Input: part model. Units: mm. Frame: model coordinates. Face numbers are marked on the shaded views. A direction names the side the tool comes from. Coordinates: 2 decimals unless noted, no trailing zeros.
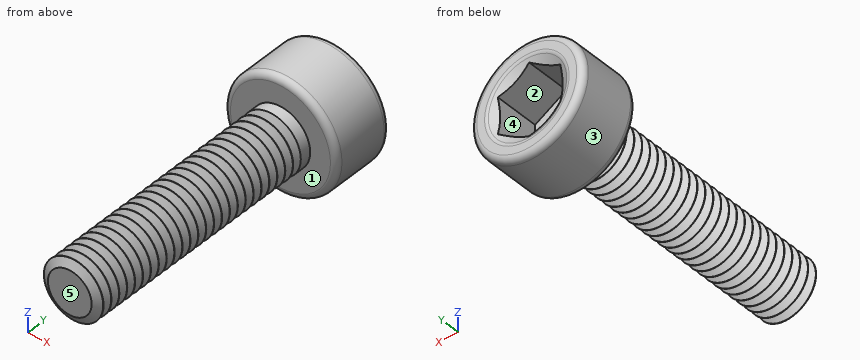
```python
from build123d import *

# Parameters (mm, degrees)
CUT_EXTRUDE1_DEPTH = 1.5
SKETCH3_R          = 1.3
CUT_EXTRUDE2_DEPTH = 1
CUT_EXTRUDE2_DRAFT = -60
FILLET1_R          = 0.2
LPATTERN1_COUNT    = 26
LPATTERN1_PITCH    = 0.3


with BuildPart() as part:
    # Sketch1 → Revolve1 (revolve)
    with BuildSketch(Plane.XY):
        with BuildLine():
            Line((0, 2), (0, -8))
            Line((0, -8), (0.95, -8))
            Line((0.95, -8), (0.95, 0))
            Line((0.95, 0), (1.6, 0))
            ThreePointArc((1.6, 0), (1.741421356, 0.058578644), (1.8, 0.2))
            Line((1.8, 0.2), (1.8, 1.8))
            ThreePointArc((1.8, 1.8), (1.741421356, 1.941421356), (1.6, 2))
            Line((1.6, 2), (0, 2))
        make_face()
    revolve(axis=Axis((0, 2, 0), (0, -1, 0)))

    # Sketch2 → Cut-Extrude1 (cut)
    with BuildSketch(Plane(origin=(0, 2, 0), x_dir=(1, 0, 0), z_dir=(0, 1, 0))):
        Polygon((1, 0.577350269), (0, 1.154700538), (-1, 0.577350269), (-1, -0.577350269), (0, -1.154700538), (1, -0.577350269), align=None)
    extrude(amount=-CUT_EXTRUDE1_DEPTH, mode=Mode.SUBTRACT)


with BuildPart() as cut_extrude2_tool:
    # Sketch3 → Cut-Extrude2 (with draft: the straight prism first)
    with BuildSketch(Plane(origin=(0, 2, 0), x_dir=(1, 0, 0), z_dir=(0, 1, 0))):
        Circle(SKETCH3_R)
    extrude(amount=-CUT_EXTRUDE2_DEPTH)
    # Cut-Extrude2: the draft: its side faces are tilted about the plane it starts from
    cut_extrude2_sides = [cut_extrude2_tool.faces().sort_by_distance(p)[0] for p in [
        (-1.3, 1.5, 0),
    ]]
    draft(cut_extrude2_sides, Plane(origin=(0, 2, 0), x_dir=(1, 0, 0), z_dir=(0, 1, 0)), CUT_EXTRUDE2_DRAFT)


with BuildPart() as part_1:
    add(part.part)

    # Cut-Extrude2: cut by cut_extrude2_tool
    add(cut_extrude2_tool.part, mode=Mode.SUBTRACT)

    # Fillet1
    fillet1_edges = [part_1.edges().sort_by_distance(p)[0] for p in [
        (-1.3, 2, 0),
    ]]
    fillet(fillet1_edges, radius=FILLET1_R)

    # Sketch4 → Cut-Revolve1 (revolve, cut)
    with BuildSketch(Plane.XY):
        Polygon((1.259807621, -7.85), (1.259807621, -8.15), (0.959807621, -8.15), (0.7, -8), (0.959807621, -7.85), align=None)
    cut_revolve1 = revolve(axis=Axis((0, 0, 0), (0, -1, 0)), mode=Mode.SUBTRACT)

    # LPattern1: Cut-Revolve1 ×26
    with Locations(*[(0, i * LPATTERN1_PITCH, 0) for i in range(1, LPATTERN1_COUNT)]):
        add(cut_revolve1, mode=Mode.SUBTRACT)


solid = part_1.part
```
Item 1: Contact query for flat-ended pins moving along their axis: P1, Ø1.5, axis at x = 0.5, y = -5, coming from the -Z side; P2, Ø0.6, axis at x = 0, z = 0.5, coming from the +Y side. Output: stop coordinate, or through.
Result:
P1: stops at z = -0.95
P2: stops at y = 0.5
Item 2: Reachability of the marked faces 4 and 5 from +Z, -Z, +X, -X, +Y, -Y: full face, straight path, thin tool, end or side. Return the list, or none.
Result:
face 4: +Y
face 5: +Z, -Z, +X, -X, -Y
Item 3: Line query: L1, parallel to Y at x = -1, z = -0.75; L2, parallel to Y at x = 0.1, z = -0.45; L3, parallel to Z at x = -0.25, y = -2.5. Output: solid intervals per line, ascending.
Result:
L1: y = 0 to 1.97
L2: y = -8 to 0.5
L3: z = -0.84 to 0.84
Item 4: Section query A-A (x = -0.85). Count the separate pieces of the cut face and the enclosed holes in it, then the cut area to 3 significant figures.
Result:
separate pieces: 26
enclosed holes: 0
area: 6.46 mm2
Item 5: Mould query, pull axis X, two halves, no side actions, for the marked faces 1, 2 and 3. Classes: +X half, -X half, draft (parallel to the pull), parting line (faces both ways), or undercut.
Result:
face 1: draft
face 2: undercut
face 3: parting line
